Input: part model. Units: mm. Frame: model coordinates. A direction names the side the tool comes from. Give positions to 0.01 mm unless a question says otherwise; leave off trailing zeros. Loops run counter-clockwise (first coordinate to the right, second up) from the corner with the lowest first, then second, coordinate; pieces in that order, holes last.
from build123d import *

# Parameters (mm, degrees)
CUT_EXTRUDE_2_DEPTH = 1.5
CHAMFER_1_SIZE      = 0.5
CUT_EXTRUDE_3_DEPTH = 4


with BuildPart() as part:
    # Эскиз1 → Повернуть1 (revolve)
    with BuildSketch(Plane.XY):
        Polygon((0, 0), (0, 2.7), (3, 2.7), (3, 1.4), (9.6, 1.4), (10, 1), (10, 0), align=None)
    revolve(axis=Axis((-1.2940953, 0, 0), (1, 0, 0)))

    # Эскиз2 → Вырез-Вытянуть2 (cut)
    with BuildSketch(Plane.ZY):
        with BuildLine():
            Line((2.632489316, 0.6), (-2.632489316, 0.6))
            ThreePointArc((-2.632489316, 0.6), (-2.7, 0), (-2.632489316, -0.6))
            Line((-2.632489316, -0.6), (2.632489316, -0.6))
            ThreePointArc((2.632489316, -0.6), (2.683069246, -0.301893066), (2.7, 0))
            ThreePointArc((2.7, 0), (2.683069246, 0.301893066), (2.632489316, 0.6))
        make_face()
    extrude(amount=-CUT_EXTRUDE_2_DEPTH, mode=Mode.SUBTRACT)

    # Фаска1
    chamfer_1_edges = [part.edges().sort_by_distance(p)[0] for p in [
        (0, -2.7, 0),
        (0, 2.110687092, 1.683745824),
    ]]
    chamfer(chamfer_1_edges, length=CHAMFER_1_SIZE)

    # Эскиз4 → Вырез-Вытянуть3 (cut, through all)
    with BuildSketch(Plane(origin=(3, 0, 0), x_dir=(0, 0, -1), z_dir=(1, 0, 0))):
        with BuildLine():
            ThreePointArc((2.271214264, 1.459995125), (1.35, 2.33826859), (0.128785736, 2.696926813))
            Line((0.128785736, 2.696926813), (2.271214264, 1.459995125))
        make_face()
        with BuildLine():
            Line((-2.271214264, 1.459995125), (-0.128785736, 2.696926813))
            ThreePointArc((-0.128785736, 2.696926813), (-1.35, 2.33826859), (-2.271214264, 1.459995125))
        make_face()
        with BuildLine():
            Line((-2.4, -1.236931688), (-2.4, 1.236931688))
            ThreePointArc((-2.4, 1.236931688), (-2.7, 0), (-2.4, -1.236931688))
        make_face()
        with BuildLine():
            Line((-0.128785736, -2.696926813), (-2.271214264, -1.459995125))
            ThreePointArc((-2.271214264, -1.459995125), (-1.35, -2.33826859), (-0.128785736, -2.696926813))
        make_face()
        with BuildLine():
            ThreePointArc((0.128785736, -2.696926813), (1.35, -2.33826859), (2.271214264, -1.459995125))
            Line((2.271214264, -1.459995125), (0.128785736, -2.696926813))
        make_face()
        with BuildLine():
            ThreePointArc((2.7, 0), (2.623928353, 0.636396103), (2.4, 1.236931688))
            Line((2.4, 1.236931688), (2.4, -1.236931688))
            ThreePointArc((2.4, -1.236931688), (2.623928353, -0.636396103), (2.7, 0))
        make_face()
    extrude(amount=-CUT_EXTRUDE_3_DEPTH, mode=Mode.SUBTRACT)


solid = part.part
(1) Reachability of faces 1 (the cylindrical face through (6.35, -1.4, 0.06)), 2 (the flat face through (1.5, 0, 0)), 3 (the flat face through (1.62, -2.087, 1.185)) from +Z, -Z, +X, -X, +Y, -Y: full face, straight path, thin tool, end or side. Return the list, or none.
Values follow:
face 1: +X
face 2: +Z, -Z, -X
face 3: +Z, +X, -X, -Y
(2) Pin query (flat end, axial travel): pin 1 Ø0.8 at (x, z) = (0.5, -0.5) entering from -Y; pin 2 Ø1.5 at (x, y) = (1.5, -1.5) entering from +Z; pin 3 Ø1.5 at (x, y) = (4, -1) entering from -Z; pin 4 Ø1 at (y, z) = (-1.5, 0.5) entering from +X. Return the tip coordinate at first contact, or that it passes through.
Values follow:
pin 1: stops at y = -2.7
pin 2: stops at z = 2.4
pin 3: stops at z = -1.38
pin 4: stops at x = 9.92
(3) Cut plane B-B (y = 0). Return the cut outline in (x, z).
Values follow:
outline: (1.5, -2.4) - (3, -2.4) - (3, -1.4) - (9.6, -1.4) - (10, -1) - (10, 1) - (9.6, 1.4) - (3, 1.4) - (3, 2.4) - (1.5, 2.4) - close
(4) Ray query, probe 1 along X at (y, z) = (0.1, -0.15); probe 2 along X at (y, z) = (0.95, 1.6); probe 3 along Z at (x, y) = (9, 0.65). Return the intervals inside material, ascending.
Values follow:
probe 1: x = 1.5 to 10
probe 2: x = 0 to 3
probe 3: z = -1.24 to 1.24
(5) Cut plane A-A (z = 0). Return the cut outline in (x, y), and give its area (3 significant figures).
Values follow:
outline: (0, -2.2) - (0.5, -2.7) - (3, -2.7) - (3, -1.4) - (9.6, -1.4) - (10, -1) - (10, 1) - (9.6, 1.4) - (3, 1.4) - (3, 2.7) - (0.5, 2.7) - (0, 2.2) - (0, 0.6) - (1.5, 0.6) - (1.5, -0.6) - (0, -0.6) - close
area: 33.6 mm2
(6) Cut plane C-C (x = 7.5). Return the cut outline in (y, z).
Values follow:
outline: circle Ø2.8 at (0, 0)
